Input: part model. Units: mm. Frame: model coordinates. Face numbers are marked on the shaded views. A direction names the side the tool comes from. Coordinates: 2 decimals unless noted, no trailing zeros. Write each loop counter-clockwise with the first axis right and the second up, starting at its lowest first coordinate (ties: lowest second). Pieces come first, ordered by that corner, then holes. Notation, with made-up numbers: (12, 72) - (63, 72) arc R32 cw to (63, 111) - close; hole circle Ø3 at (6, 82). An arc over 180 degrees is marked (long way). One line per question, with ' | ' between items. Start each with the question number.
1) Section query C-C on y = -66. Return loops of the section in (x, z), and give its area (3 significant figures).
2) Section query D-D on x = 46. Return loops of the section in (y, z), and give its area (3 significant figures).
3) Reachability of the marked faces 1, 2 and 3 from +Z, -Z, +X, -X, +Y, -Y: full face, straight path, thin tool, end or side. Return the list, or none.
4) Line query: line 1 (Y direction, x = 43, z = 19); line 2 (Y direction, x = -80, z = 14); line 3 (Z direction, x = -14, y = 11). Output: solid intervals per line, ascending.
5) First-contact query: P1, Ø12.5, axis at x = -78.5, z = 9.5, coming from the -Y side; P2, Ø7.5, axis at x = -9, z = 17.5, coming from the -Y side (3 decimals); P3, Ø1.5, axis at y = -83.5, z = 3, coming from the -X side (3 decimals). Flat tips, straight axial feed; report the tip coordinate or a pass-through.
6) Section query B-B on z = 18.5. Give the number of separate pieces and of enclosed holes in the cut face, and give its area (3 significant figures).
7) Section query A-A on x = -104.5. Return loops of the section in (y, z).
```python
from build123d import *

# Parameters (mm, degrees)
F0_W     = 300
F0_H     = 300
F1_DEPTH = 25
F3_DEPTH = 25
F4_R     = 20
F5_R     = 5


with BuildPart() as f1:
    # F0 (on Top) → F1 (new body)
    with BuildSketch(Plane.XY):
        Rectangle(F0_W, F0_H)
    extrude(amount=-F1_DEPTH)

    # F2 (on face) → F3 (join)
    with BuildSketch(Plane.XY):
        with BuildLine():
            ThreePointArc((-37.5, -30.156865), (-20.039255, -51.252458), (-40, -70))
            Line((-40, -70), (-90, -70))
            Line((-90, -70), (-110, -110))
            Line((-110, -110), (-40, -110))
            ThreePointArc((-40, -110), (19.882236, -53.757375), (-32.5, 9.529404))
            ThreePointArc((-32.5, 9.529404), (-49.960745, 30.624998), (-30, 49.372539))
            Line((-30, 49.372539), (10, 49.372539))
            ThreePointArc((10, 49.372539), (68.471551, 65.713145), (110, 110))
            ThreePointArc((110, 110), (71.308268, 94.61238), (30, 89.372539))
            Line((30, 89.372539), (-30, 89.372539))
            ThreePointArc((-30, 89.372539), (-89.882236, 33.129914), (-37.5, -30.156865))
        make_face()
        with BuildLine():
            ThreePointArc((100, 75.721052), (58.914743, 47.359298), (10, 37.372539))
            ThreePointArc((10, 37.372539), (-4.817424, 26.491687), (1.128978, 9.096592))
            ThreePointArc((1.128978, 9.096592), (7.932224, 3.726175), (14.040846, -2.422832))
            ThreePointArc((14.040846, -2.422832), (73.830182, 18.158186), (100, 75.721052))
        make_face()
        with BuildLine():
            ThreePointArc((85, 12.229434), (56.413934, -7.140348), (22.700465, -14.60718))
            ThreePointArc((22.700465, -14.60718), (30.620541, -35.973627), (31.466948, -58.745018))
            ThreePointArc((31.466948, -58.745018), (66.554074, -29.533671), (85, 12.229434))
        make_face()
        with BuildLine():
            ThreePointArc((28.093718, -73.39328), (16.967091, -94.031245), (-0.200503, -110))
            ThreePointArc((-0.200503, -110), (44.30119, -92.515885), (65, -49.415372))
            ThreePointArc((65, -49.415372), (47.736246, -63.235005), (28.093718, -73.39328))
        make_face()
    extrude(amount=F3_DEPTH)

    # F4
    f4_edges = [f1.edges().sort_by_distance(p)[0] for p in [
        (14.040846, -2.422832, 12.5),
        (28.093718, -73.39328, 12.5),
    ]]
    fillet(f4_edges, radius=F4_R)

    # F5
    f5_edges = [f1.edges().sort_by_distance(p)[0] for p in [
        (22.700465, -14.60718, 12.5),
        (31.466948, -58.745018, 12.5),
        (-0.200503, -110, 12.5),
    ]]
    fillet(f5_edges, radius=F5_R)


solid = f1.part
```
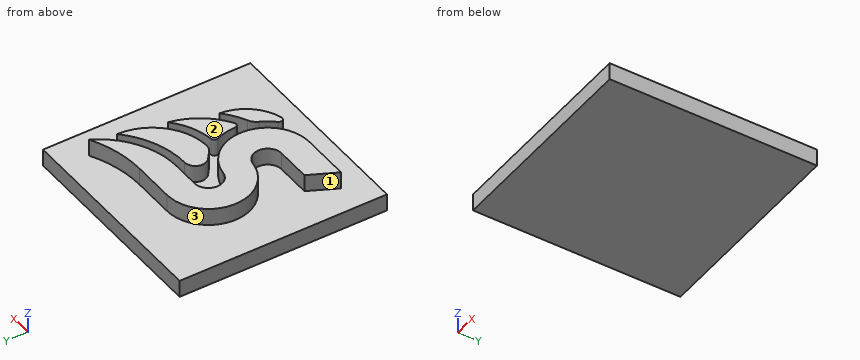
Answer key:
1) outline: (-150, -25) - (150, -25) - (150, 0) - (61.58, 0) - (61.58, 25) - (43.25, 25) - (43.25, 0) - (17.83, 0) - (17.83, 25) - (-28, 25) - (-28, 0) - (-150, 0) - close | area: 9,100 mm²
2) outline: (-150, -25) - (150, -25) - (150, 0) - (90.15, 0) - (90.15, 25) - (55.27, 25) - (55.27, 0) - (42.68, 0) - (42.68, 25) - (1.69, 25) - (1.69, 0) - (-10.9, 0) - (-10.9, 25) - (-49.85, 25) - (-49.85, 0) - (-64.34, 0) - (-64.34, 25) - (-90.88, 25) - (-90.88, 0) - (-150, 0) - close | area: 11,000 mm²
3) face 1: +Z, -X, +Y | face 2: +Z, +X, -X, +Y, -Y | face 3: +Z, -X
4) line 1: -93.69 to -66.15, -51.97 to -11.73, 0.73 to 41.82, 54.31 to 89.88 | line 2: -110 to -70, -3.79 to 62.54 | line 3: -25 to 0
5) P1: y = -110 | P2: y = -103.455 | P3: x = -97.125
6) separate pieces: 4 | enclosed holes: 0 | area: 23,000 mm²
7) outline: (-150, -25) - (150, -25) - (150, 0) - (-99, 0) - (-99, 25) - (-110, 25) - (-110, 0) - (-150, 0) - close
